from build123d import *

# Parameters (mm, degrees)
SKETCH1_W           = 60
SKETCH1_H           = 90
BOSS_EXTRUDE1_DEPTH = 4.7625
FILLET1_R           = 5
SKETCH2_R           = 1.7
CUT_EXTRUDE1_DEPTH  = 5
CUT_EXTRUDE2_DEPTH  = 3


with BuildPart() as part:
    # Sketch1 → Boss-Extrude1 (new body)
    with BuildSketch(Plane.XY):
        Rectangle(SKETCH1_W, SKETCH1_H)
    extrude(amount=BOSS_EXTRUDE1_DEPTH)

    # Fillet1
    fillet1_edges = [part.edges().sort_by_distance(p)[0] for p in [
        (-30, 45, 2.38125),
        (30, 45, 2.38125),
        (30, -45, 2.38125),
        (-30, -45, 2.38125),
    ]]
    fillet(fillet1_edges, radius=FILLET1_R)

    # Sketch2 → Cut-Extrude1 (cut)
    with BuildSketch(Plane.XY):
        with Locations((-25, 40)):
            Circle(SKETCH2_R)
        with Locations((25, 40)):
            Circle(SKETCH2_R)
        with Locations((25, -40)):
            Circle(SKETCH2_R)
        with Locations((-25, -40)):
            Circle(SKETCH2_R)
    extrude(amount=CUT_EXTRUDE1_DEPTH, mode=Mode.SUBTRACT)

    # Sketch3 → Cut-Extrude2 (cut)
    with BuildSketch(Plane.XY):
        Polygon((-23.383419246, 37.2), (-21.766838493, 40), (-23.383419246, 42.8), (-26.616580754, 42.8), (-28.233161507, 40), (-26.616580754, 37.2), align=None)
        Polygon((26.616580754, 37.2), (28.233161507, 40), (26.616580754, 42.8), (23.383419246, 42.8), (21.766838493, 40), (23.383419246, 37.2), align=None)
        Polygon((26.616580754, -42.8), (28.233161507, -40), (26.616580754, -37.2), (23.383419246, -37.2), (21.766838493, -40), (23.383419246, -42.8), align=None)
        Polygon((-23.383419246, -42.8), (-21.766838493, -40), (-23.383419246, -37.2), (-26.616580754, -37.2), (-28.233161507, -40), (-26.616580754, -42.8), align=None)
    extrude(amount=CUT_EXTRUDE2_DEPTH, mode=Mode.SUBTRACT)


solid = part.part
Could you check a few things on this model? Use its own coordinates, in mm. A direction names the side the tool comes from. Give positions to 0.01 mm unless a question says otherwise; leave off trailing zeros. Return JSON: item names as keys, results as strings. Group by question number.
Q1. Suppose I cut it at A-A, the plane z = 2.15. State how many separate pieces and enclosed holes the cut face has, and give its area (3 significant figures).
Q2. Thinking about a two-plate mould opening in Y: for faces 1 (the face through (-22.586, -41.42, 1.479)), 2 (the face through (-29, 43, 2)), 3 (the face through (0, -45, 2)), which applies, pulls with the +Y half, pulls with the -Y half, needs draft (parallel to the pull), parting line crosses it, or undercut?
Q3. Please list where these lines run through material, in increasing order: line 1 along X through (y, z) = (-40, 3.95); line 2 along Y through (x, z) = (25, 1.1); line 3 along Y through (x, z) = (-25, 3.5). Write a range as [from, to].
Q4. Which directions (+Z, -Z, +X, -X, +Y, -Y) give clear straight access to the entire face, cutting with the end or side of a thin tool? Please do faces 4 (the face through (-24.2, 38.5, 3.9)), 5 (the face through (-27.414, 41.42, 1.479)).
Q5. Will these pins go through, and if not, where does the flat tip stop? pin 1 Ø3 at (x, y) = (25, -40) entering from +Z; pin 2 Ø1.7 at (x, y) = (-25.5, 41) entering from -Z.
Resolved:
{
 "1": {"separate pieces": "1", "enclosed holes": "4", "area": "5,270 mm2"},
 "2": {"face 1": "undercut", "face 2": "pulls with the +Y half", "face 3": "pulls with the -Y half"},
 "3": {"line 1": "x = [-30, -26.7], [-23.3, 23.3], [26.7, 30]", "line 2": "y = [-45, -42.8], [-37.2, 37.2], [42.8, 45]", "line 3": "y = [-45, -41.7], [-38.3, 38.3], [41.7, 45]"},
 "4": {"face 4": "+Z, -Z", "face 5": "-Z"},
 "5": {"pin 1": "passes through", "pin 2": "stops at z = 3"}
}
